```python
from build123d import *

# Parameters (mm, degrees)
SKETCH_1_R          = 1.5
EXTRUDE_1_DEPTH     = 3
SKETCH_2_W          = 7
SKETCH_2_H          = 7
CUT_EXTRUDE_1_DEPTH = 1.5
SKETCH_3_R          = 3.5
CUT_EXTRUDE_2_DEPTH = 3
CUT_EXTRUDE_3_DEPTH = 3


with BuildPart() as part:
    # 草图1 → 凸台-拉伸1 (new body)
    with BuildSketch(Plane.XY):
        with BuildLine():
            Line((3, 0), (68, 0))
            ThreePointArc((68, 0), (70.121320344, -0.878679656), (71, -3))
            Line((71, -3), (71, -23.6))
            ThreePointArc((71, -23.6), (70.121320344, -25.721320344), (68, -26.6))
            Line((68, -26.6), (3, -26.6))
            ThreePointArc((3, -26.6), (0.878679656, -25.721320344), (0, -23.6))
            Line((0, -23.6), (0, -3))
            ThreePointArc((0, -3), (0.878679656, -0.878679656), (3, 0))
        make_face()
        with Locations((3, -3)):
            Circle(SKETCH_1_R, mode=Mode.SUBTRACT)
        with Locations((68, -3)):
            Circle(SKETCH_1_R, mode=Mode.SUBTRACT)
        with Locations((68, -23.6)):
            Circle(SKETCH_1_R, mode=Mode.SUBTRACT)
        with Locations((3, -23.6)):
            Circle(SKETCH_1_R, mode=Mode.SUBTRACT)
    extrude(amount=EXTRUDE_1_DEPTH)

    # 草图2 → 切除-拉伸1 (cut)
    with BuildSketch(Plane.XY.offset(3)):
        with Locations((15.5, -16.6)):
            Rectangle(SKETCH_2_W, SKETCH_2_H)
        with Locations((28.833, -16.6)):
            Rectangle(SKETCH_2_W, SKETCH_2_H)
        with Locations((42.166, -16.6)):
            Rectangle(SKETCH_2_W, SKETCH_2_H)
        with Locations((55.5, -16.6)):
            Rectangle(SKETCH_2_W, SKETCH_2_H)
    extrude(amount=-CUT_EXTRUDE_1_DEPTH, mode=Mode.SUBTRACT)

    # 草图3 → 切除-拉伸2 (cut)
    with BuildSketch(Plane.XY.offset(3)):
        with Locations((15.487336513, -16.581748308)):
            Circle(SKETCH_3_R)
        with Locations((28.821952613, -16.591607422)):
            Circle(SKETCH_3_R)
        with Locations((42.164313749, -16.595901173)):
            Circle(SKETCH_3_R)
        with Locations((55.50458657, -16.602564336)):
            Circle(SKETCH_3_R)
    extrude(amount=-CUT_EXTRUDE_2_DEPTH, mode=Mode.SUBTRACT)

    # 草图4 → 切除-拉伸3 (cut)
    with BuildSketch(Plane(origin=(0, 0, 0), x_dir=(-1, 0, 0), z_dir=(0, 0, -1))):
        Polygon((-41.586971982, -4), (-51.880305316, -4), (-53, -9), (-42.706666667, -9), align=None)
        with BuildLine():
            Line((-53.380305316, -4), (-59.5, -4))
            ThreePointArc((-59.5, -4), (-60.207106781, -4.292893219), (-60.5, -5))
            Line((-60.5, -5), (-60.5, -8))
            ThreePointArc((-60.5, -8), (-60.207106781, -8.707106781), (-59.5, -9))
            Line((-59.5, -9), (-54.5, -9))
            Line((-54.5, -9), (-53.380305316, -4))
        make_face()
        Polygon((-29.79, -4), (-40.086971982, -4), (-41.206666667, -9), (-30.909694684, -9), align=None)
        Polygon((-18, -4), (-28.29, -4), (-29.409694684, -9), (-19.119694684, -9), align=None)
        with BuildLine():
            Line((-11.5, -4), (-16.5, -4))
            Line((-16.5, -4), (-17.619694684, -9))
            Line((-17.619694684, -9), (-11.5, -9))
            ThreePointArc((-11.5, -9), (-10.792893219, -8.707106781), (-10.5, -8))
            Line((-10.5, -8), (-10.5, -5))
            ThreePointArc((-10.5, -5), (-10.792893219, -4.292893219), (-11.5, -4))
        make_face()
    extrude(amount=-CUT_EXTRUDE_3_DEPTH, mode=Mode.SUBTRACT)


solid = part.part
```
The model under review builds one solid part; all positions refer to its coordinate system, in mm. A direction names the side the tool comes from. Give positions to 0.01 mm unless a question says otherwise; leave off trailing zeros.
(1) For P1, Ø2.5, axis at x = 57.5, y = -18.5, coming from the +Z side, flat-tipped, find the tip position at first contact; note if it passes through.
(2) Tool access review of faces 1 (the flat face through (36, -13, 0)), 2 (the flat face through (27, -13.1, 2)), 3 (the flat face through (60.5, -6, 1)): name each direction out of +Z, -Z, +X, -X, +Y, -Y from which nothing blocks a thin tool from reaching the whole face with its end or side.
(3) Consider section A-A, the plane z = 2.35. Give the number of separate pieces and of enclosed holes in the cut face, and give its area (3 significant figures).
(4) To check wall thickness, follow L1, parallel to Y at x = 68, z = 2.1; L2, parallel to X at y = -14.5, z = 2.8; L3, parallel to Y at x = 58.5, z = 2.15. State the ranges of each line that lie inside material, in increasing order.
Returned:
1. P1: stops at z = 1.5
2. face 1: -Z, +X, -X, +Y, -Y
2. face 2: +Z
2. face 3: +Z, -Z
3. separate pieces: 1
3. enclosed holes: 13
3. area: 1,440 mm2
4. L1: y = -26.6 to -25.1, -22.1 to -4.5, -1.5 to 0
4. L2: x = 0 to 12, 19 to 25.33, 32.33 to 38.67, 45.67 to 52, 59 to 71
4. L3: y = -26.6 to -20.1, -13.1 to -9, -4 to 0
